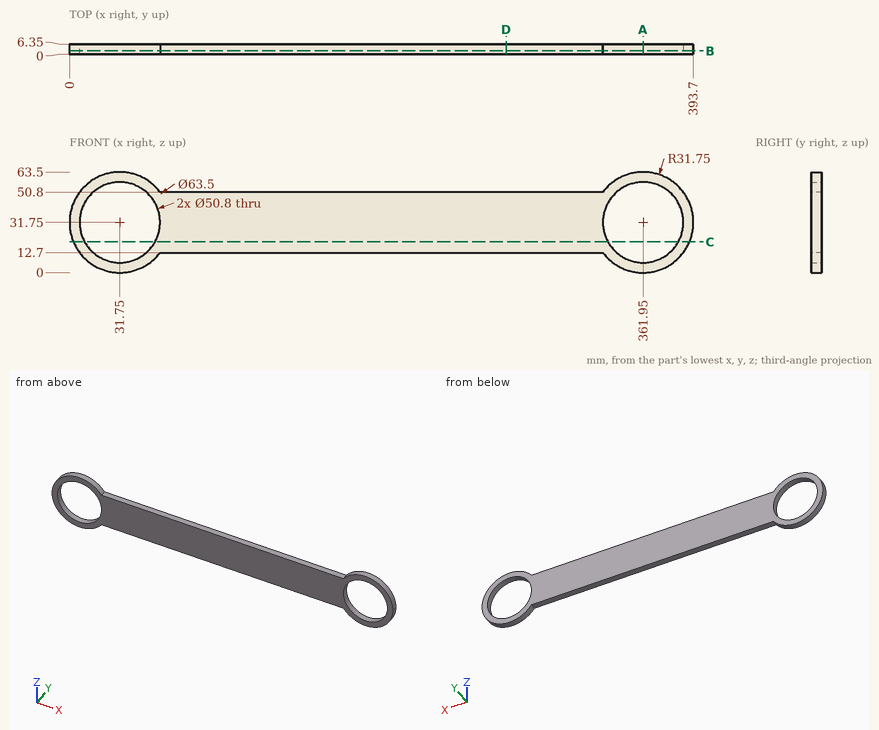
Input: dimensioned drawing with shaded views. Units: mm. Origin: part minimum x, y, z. Round coordinates to 2 decimals unless told otherwise and drop trailing zeros. Order: outer loops, then holes, each group sorted by start corner. A loop starts at its lowest first (then second) coordinate and runs counter-clockwise, first axis right, second up.
1. Material intervals for line 1 (X direction, y = 5.5, z = 30); line 2 (X direction, y = 1.25, z = 31.5); line 3 (Z direction, x = 31.75, y = 5), sorted ascending.
The answers:
line 1: x = 0.05 to 6.41, 57.09 to 336.61, 387.29 to 393.65
line 2: x = 0 to 6.35, 57.15 to 336.55, 387.35 to 393.7
line 3: z = 0 to 6.35, 57.15 to 63.5
2. Cut plane D-D, the plane x = 275.5. Output: boundary loops of the cut face in (y, z).
The answers:
outline: (0, 12.7) - (6.35, 12.7) - (6.35, 50.8) - (0, 50.8) - close
3. Cut plane C-C, the plane z = 19.5. Output: boundary loops of the cut face in (x, y).
The answers:
outline: (2.46, 0) - (9.5, 0) - (9.5, 6.35) - (2.46, 6.35) - close; (54, 0) - (339.7, 0) - (339.7, 6.35) - (54, 6.35) - close; (384.2, 0) - (391.24, 0) - (391.24, 6.35) - (384.2, 6.35) - close
4. Cut plane A-A, the plane x = 361.95. Output: boundary loops of the cut face in (y, z), then the cut area to 3 significant figures.
The answers:
outline: (0, 0) - (6.35, 0) - (6.35, 6.35) - (0, 6.35) - close; (0, 57.15) - (6.35, 57.15) - (6.35, 63.5) - (0, 63.5) - close
area: 80.6 mm2
5. Cut plane B-B, the plane y = 2. Output: boundary loops of the cut face in (x, z), then the cut area to 3 significant figures.
The answers:
outline: (57.15, 12.7) - (336.55, 12.7) arc R31.75 ccw (long way) to (336.55, 50.8) - (57.15, 50.8) arc R31.75 ccw (long way) to start; hole circle Ø50.8 at (31.75, 31.75); hole circle Ø50.8 at (361.95, 31.75)
area: 12,600 mm2
6. Pin query (flat end, axial travel): P1, Ø3, axis at y = 1, z = 24.5, coming from the -X side (3 decimals). Return the tip coordinate at first contact, or that it passes through.
The answers:
P1: stops at x = 0.525
